Here's the drawing with two shaded views (mm, measured from the low corner). I have some questions. A direction names the side the tool comes from. Round coordinates to 2 decimals unless told otherwise and drop trailing zeros. Order: outer loops, then holes, each group sorted by start corner. A loop starts at its lowest first (then second) coordinate and runs counter-clockwise, first axis right, second up. Notation, with made-up numbers: (53.25, 46.25) -> (98.25, 46.25) arc R19 cw to (98.25, 56.25) -> close; hole circle Ø2 at (18, -36). An arc over 180 degrees is marked (long way). One line per question, with ' | ' between items.
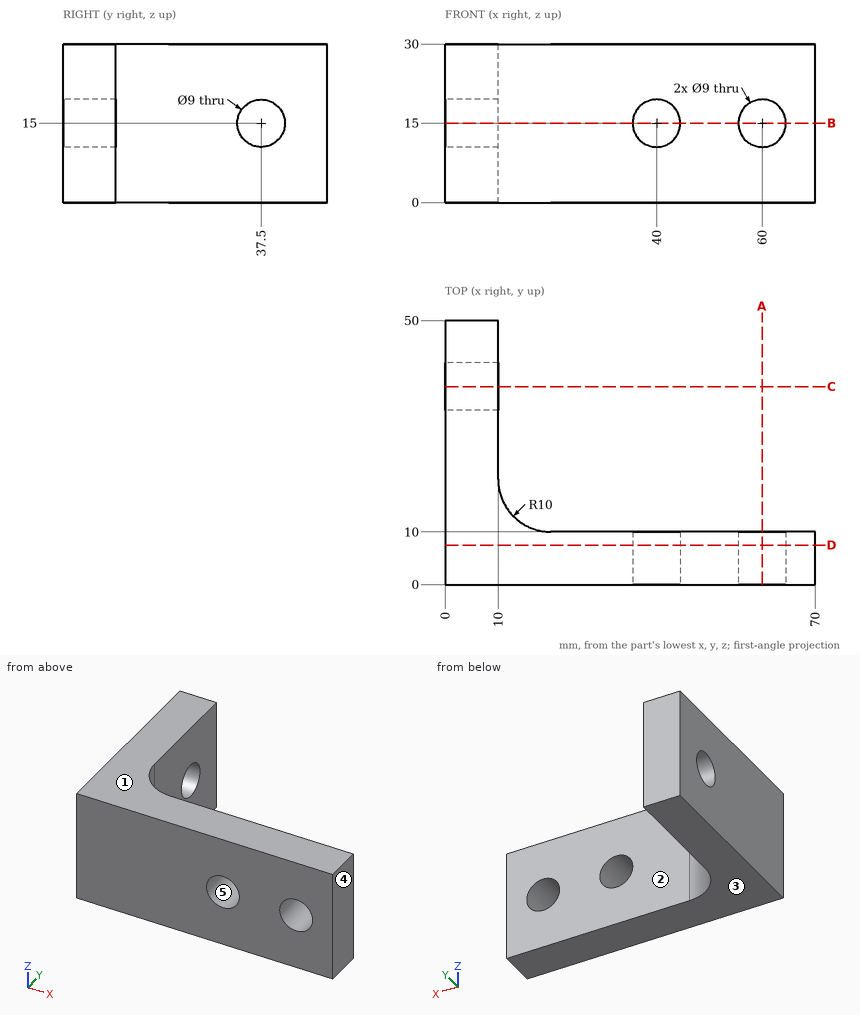
1. I want a section at B-B on z = 15. List the corners of the cut face in (x, y) for me.
From the geometry:
outline: (0, 0) -> (35.5, 0) -> (35.5, 10) -> (20, 10) arc R10 cw to (10, 20) -> (10, 33) -> (0, 33) -> close; (0, 42) -> (10, 42) -> (10, 50) -> (0, 50) -> close; (44.5, 0) -> (55.5, 0) -> (55.5, 10) -> (44.5, 10) -> close; (64.5, 0) -> (70, 0) -> (70, 10) -> (64.5, 10) -> close
2. On a 3-axis mill with a long thin cutter (end or side, diameter ignored), from which of +Z, -Z, +X, -X, +Y, -Y can I reach the whole of each face in a straight line? I mean the marked faces 1 and 2. Say none if no direction works.
From the geometry:
face 1: +Z, +X, -X, +Y, -Y | face 2: +Z, -Z, +X, +Y
3. I need wall thicknesses on probe 1 along Z at (x, y) = (40, 2); probe 2 along Y at (x, z) = (3.75, 15); probe 3 along Y at (x, z) = (40, 5). Which ranges of each line are inside material? Lowest first, please.
From the geometry:
probe 1: z = 0 to 10.5, 19.5 to 30 | probe 2: y = 0 to 33, 42 to 50 | probe 3: y = 0 to 10
4. I want a section at A-A on x = 60. List the corners of the cut face in (y, z) for me.
From the geometry:
outline: (0, 0) -> (10, 0) -> (10, 10.5) -> (0, 10.5) -> close; (0, 19.5) -> (10, 19.5) -> (10, 30) -> (0, 30) -> close
5. If we mould it in two halves opening along X, with no side actions, what happens to the marked faces 3, 4 and 5? For each: pulls with the +X half, pulls with the -X half, needs draft (parallel to the pull), parting line crosses it, or undercut.
From the geometry:
face 3: needs draft | face 4: pulls with the +X half | face 5: undercut
6. I want a section at D-D on y = 7.5. List the corners of the cut face in (x, z) for me.
From the geometry:
outline: (0, 0) -> (70, 0) -> (70, 30) -> (0, 30) -> close; hole circle Ø9 at (40, 15); hole circle Ø9 at (60, 15)
7. I'm going to push flat-ended pins straight in: pin 1 (6 mm diameter, centred on x = 61, z = 26, fed in from +Y); pin 2 (3 mm diameter, centred on y = 18.5, z = 7, fed in from +X); pin 3 (8 mm diameter, centred on y = 37.5, z = 15, fed in from -X); pin 4 (9 mm diameter, centred on y = 32.5, z = 18, fed in from +X). Where does each tip first touch, or does it pass through?
From the geometry:
pin 1: stops at y = 10 | pin 2: stops at x = 10.46 | pin 3: passes through | pin 4: stops at x = 10
